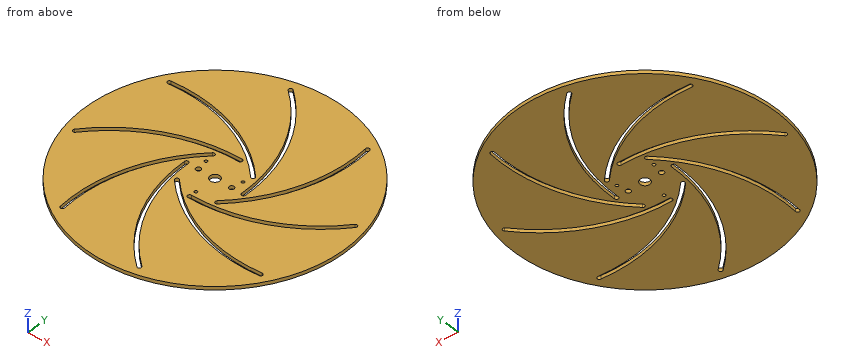
from build123d import *

# Parameters (mm, degrees)
SKETCH1_R                = 135
SKETCH1_R_2              = 5
SKETCH1_R_3              = 2.5
SKETCH1_R_4              = 1.5
BOSS_EXTRUDE1_DEPTH      = 1.75
BOSS_EXTRUDE1_DEPTH_BACK = 1.75


with BuildPart() as part:
    # Sketch1 → Boss-Extrude1 (new body, two sides)
    with BuildSketch(Plane.XY) as boss_extrude1_sk:
        Circle(SKETCH1_R)
        Circle(SKETCH1_R_2, mode=Mode.SUBTRACT)
        with Locations((-17.5, 0)):
            Circle(SKETCH1_R_3, mode=Mode.SUBTRACT)
        with Locations((17.5, 0)):
            Circle(SKETCH1_R_3, mode=Mode.SUBTRACT)
        with Locations((0, -22.5)):
            Circle(SKETCH1_R_4, mode=Mode.SUBTRACT)
        with Locations((-19.485571585, 11.25)):
            Circle(SKETCH1_R_4, mode=Mode.SUBTRACT)
        with Locations((19.485571585, 11.25)):
            Circle(SKETCH1_R_4, mode=Mode.SUBTRACT)
        with BuildLine():
            ThreePointArc((0, 32), (-68.434713414, 16.3), (-123.182484144, -27.66))
            ThreePointArc((-123.182484144, -27.66), (-122.853280525, -30.46920362), (-120.044076905, -30.14))
            ThreePointArc((-120.044076905, -30.14), (-66.691153836, 12.7), (0, 28))
            ThreePointArc((0, 28), (2, 30), (0, 32))
        make_face(mode=Mode.SUBTRACT)
        with BuildLine():
            ThreePointArc((22.627416998, 22.627416998), (-36.86480939, 59.916490457), (-106.66174343, 67.544596294))
            ThreePointArc((-106.66174343, 67.544596294), (-108.415368247, 65.325407253), (-106.196179206, 63.571782436))
            ThreePointArc((-106.196179206, 63.571782436), (-38.177511002, 56.138023244), (19.798989873, 19.798989873))
            ThreePointArc((19.798989873, 19.798989873), (22.627416998, 19.798989873), (22.627416998, 22.627416998))
        make_face(mode=Mode.SUBTRACT)
        with BuildLine():
            ThreePointArc((32, 0), (16.3, 68.434713414), (-27.66, 123.182484144))
            ThreePointArc((-27.66, 123.182484144), (-30.46920362, 122.853280525), (-30.14, 120.044076905))
            ThreePointArc((-30.14, 120.044076905), (12.7, 66.691153836), (28, 0))
            ThreePointArc((28, 0), (30, -2), (32, 0))
        make_face(mode=Mode.SUBTRACT)
        with BuildLine():
            ThreePointArc((22.627416998, -22.627416998), (59.916490457, 36.86480939), (67.544596294, 106.66174343))
            ThreePointArc((67.544596294, 106.66174343), (65.325407253, 108.415368247), (63.571782436, 106.196179206))
            ThreePointArc((63.571782436, 106.196179206), (56.138023244, 38.177511002), (19.798989873, -19.798989873))
            ThreePointArc((19.798989873, -19.798989873), (19.798989873, -22.627416998), (22.627416998, -22.627416998))
        make_face(mode=Mode.SUBTRACT)
        with BuildLine():
            ThreePointArc((0, -32), (68.434713414, -16.3), (123.182484144, 27.66))
            ThreePointArc((123.182484144, 27.66), (122.853280525, 30.46920362), (120.044076905, 30.14))
            ThreePointArc((120.044076905, 30.14), (66.691153836, -12.7), (0, -28))
            ThreePointArc((0, -28), (-2, -30), (0, -32))
        make_face(mode=Mode.SUBTRACT)
        with BuildLine():
            ThreePointArc((-22.627416998, -22.627416998), (36.86480939, -59.916490457), (106.66174343, -67.544596294))
            ThreePointArc((106.66174343, -67.544596294), (108.415368247, -65.325407253), (106.196179206, -63.571782436))
            ThreePointArc((106.196179206, -63.571782436), (38.177511002, -56.138023244), (-19.798989873, -19.798989873))
            ThreePointArc((-19.798989873, -19.798989873), (-22.627416998, -19.798989873), (-22.627416998, -22.627416998))
        make_face(mode=Mode.SUBTRACT)
        with BuildLine():
            ThreePointArc((-32, 0), (-16.3, -68.434713414), (27.66, -123.182484144))
            ThreePointArc((27.66, -123.182484144), (30.46920362, -122.853280525), (30.14, -120.044076905))
            ThreePointArc((30.14, -120.044076905), (-12.7, -66.691153836), (-28, 0))
            ThreePointArc((-28, 0), (-30, 2), (-32, 0))
        make_face(mode=Mode.SUBTRACT)
        with BuildLine():
            ThreePointArc((-22.627416998, 22.627416998), (-59.916490457, -36.86480939), (-67.544596294, -106.66174343))
            ThreePointArc((-67.544596294, -106.66174343), (-65.325407253, -108.415368247), (-63.571782436, -106.196179206))
            ThreePointArc((-63.571782436, -106.196179206), (-56.138023244, -38.177511002), (-19.798989873, 19.798989873))
            ThreePointArc((-19.798989873, 19.798989873), (-19.798989873, 22.627416998), (-22.627416998, 22.627416998))
        make_face(mode=Mode.SUBTRACT)
    extrude(amount=BOSS_EXTRUDE1_DEPTH)
    extrude(boss_extrude1_sk.sketch, amount=-BOSS_EXTRUDE1_DEPTH_BACK)


solid = part.part
Check sheet for the modelled part. Datum: model origin and axes. Units: mm. Round coordinates to 2 decimals unless told otherwise and drop trailing zeros. Order: outer loops, then holes, each group sorted by start corner. A loop starts at its lowest first (then second) coordinate and runs counter-clockwise, first axis right, second up. Notation, with made-up numbers: M 23,-39 L 50,-39 A26 ccw 50,-18 Z; hole C 64.5,-13 d5. An arc over 180 degrees is marked long. One line per item, written item: value. Start each with the question number.
1. Section check B-B on x = -9. Enter the section's corners in (y, z).
2. Section check A-A on y = -81.5. Enter the section's corners in (x, z), and give its area (3 significant figures).
3. Gauge pin test, flat end, axial feed: P1, Ø8, axis at x = 0, y = 0, coming from the +Z side. Record the tip position at first contact, or that the pin passes through.
4. Scan lines: line 1 along Y through (x, z) = (7, -1.35); line 2 along Y through (x, z) = (105, 0.1); line 3 along Y through (x, z) = (90, 1.05). Record each from-to range of solid material in increasing order.
Results found:
1. outline: M -134.7,-1.75 L -81.81,-1.75 L -81.81,1.75 L -134.7,1.75 Z; M -73.84,-1.75 L -34.76,-1.75 L -34.76,1.75 L -73.84,1.75 Z; M -29.61,-1.75 L 27.74,-1.75 L 27.74,1.75 L -29.61,1.75 Z; M 31.74,-1.75 L 42.4,-1.75 L 42.4,1.75 L 31.74,1.75 Z; M 47.06,-1.75 L 99.76,-1.75 L 99.76,1.75 L 47.06,1.75 Z; M 105.8,-1.75 L 134.7,-1.75 L 134.7,1.75 L 105.8,1.75 Z
2. outline: M -107.62,-1.75 L -68.46,-1.75 L -68.46,1.75 L -107.62,1.75 Z; M -64.46,-1.75 L -9.19,-1.75 L -9.19,1.75 L -64.46,1.75 Z; M -4.49,-1.75 L 107.62,-1.75 L 107.62,1.75 L -4.49,1.75 Z
2. area: 723 mm^2
3. P1: through
4. line 1: -134.82 to -103.56, -97.39 to -45.87, -41.17 to -31.84, -27.84 to 31.24, 36.31 to 77.36, 85 to 134.82
4. line 2: -84.85 to -67.73, -63.71 to 8.28, 13.72 to 84.85
4. line 3: -100.62 to -68.6, -64.6 to -3.64, 1.27 to 100.62
